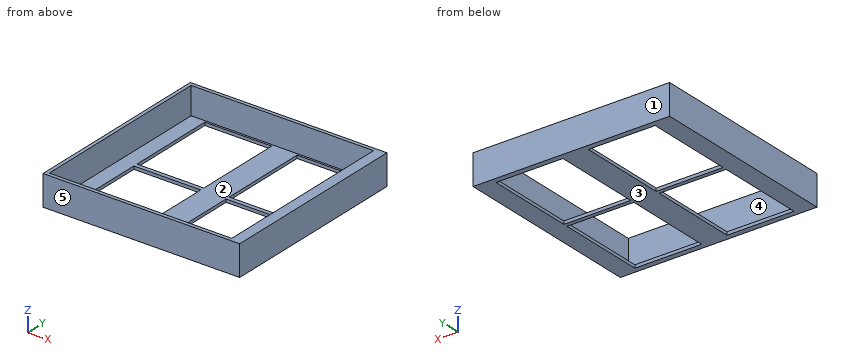
from build123d import *

# Parameters (mm, degrees)
SKETCH_W                        = 194
SKETCH_H                        = 191
PAD_DEPTH                       = 30
SKETCH001_W                     = 180
SKETCH001_H                     = 184
POCKET_DEPTH                    = 27
SKETCH002_W                     = 66
SKETCH002_H                     = 88
POCKET001_DEPTH                 = 5
SKETCH002_LINEARPATTERN_2_W     = 66
SKETCH002_LINEARPATTERN_2_H     = 88
POCKET001_LINEARPATTERN_2_DEPTH = 5
LINEARPATTERN001_COUNT          = 2
LINEARPATTERN001_PITCH          = 92


with BuildPart() as part:
    # Sketch → Pad (new body)
    with BuildSketch(Plane.XY):
        with Locations((97, 95.5)):
            Rectangle(SKETCH_W, SKETCH_H)
    extrude(amount=PAD_DEPTH)

    # Sketch001 (on Face6 of Pad) → Pocket (cut)
    with BuildSketch(Plane.XY.offset(30)):
        with Locations((93.5, 95.5)):
            Rectangle(SKETCH001_W, SKETCH001_H)
    extrude(amount=-POCKET_DEPTH, mode=Mode.SUBTRACT)

    # Sketch002 (on Face11 of Pocket) → Pocket001 (cut)
    with BuildSketch(Plane.XY.offset(3)):
        with Locations((51.5, 141.5)):
            Rectangle(SKETCH002_W, SKETCH002_H)
    pocket001 = extrude(amount=-POCKET001_DEPTH, mode=Mode.SUBTRACT)

    # Sketch002 LinearPattern 2 → Pocket001 LinearPattern 2 (cut)
    with BuildSketch(Plane(origin=(91, 0, 3), x_dir=(1, 0, 0), z_dir=(0, 0, 1))):
        with Locations((51.5, 141.5)):
            Rectangle(SKETCH002_LINEARPATTERN_2_W, SKETCH002_LINEARPATTERN_2_H)
    pocket001_linearpattern_2 = extrude(amount=-POCKET001_LINEARPATTERN_2_DEPTH, mode=Mode.SUBTRACT)

    # LinearPattern001: Pocket001, Pocket001 LinearPattern 2 ×2
    with Locations(*[(0, -i * LINEARPATTERN001_PITCH, 0) for i in range(1, LINEARPATTERN001_COUNT)]):
        add(pocket001, mode=Mode.SUBTRACT)
        add(pocket001_linearpattern_2, mode=Mode.SUBTRACT)


solid = part.part
Check sheet for the modelled part. Datum: model origin and axes. Units: mm. Face numbers are marked on the shaded views. A direction names the side the tool comes from. Round coordinates to 2 decimals unless told otherwise and drop trailing zeros. Write each loop counter-clockwise with the first axis right and the second up, starting at its lowest first coordinate (ties: lowest second). Pieces come first, ordered by that corner, then holes. Notation, with made-up numbers: (75.25, -19) -> (121.25, -19) arc R21 cw to (121.25, 7) -> close; hole circle Ø7 at (81.25, -12). An arc over 180 degrees is marked (long way). Answer as CSV lines item,"result". Start each with the question number.
1) Release check for a two-part mould opening along Y. For the marked faces 1, 2 and 3 record: pulls with the +Y half, pulls with the -Y half, needs draft (parallel to the pull), parting line crosses it, or undercut.
2) Material ranges on line 1 (X direction, y = 118, z = 20.75); line 2 (Y direction, x = 158, z = 6); line 3 (Z direction, x = 179.5, y = 67), recorded low to high. Write a range as from..to.
3) Tool access check on the marked faces 4 and 5. Record the directions out of +Z, -Z, +X, -X, +Y, -Y that give a thin tool (end or side, any length) a straight path to the whole face; none if there is none.
4) Section check B-B on x = 75. Enter the section's corners in (y, z), and give its area (3 significant figures).
5) Section check C-C on z = 6.25. Enter the section's corners in (x, y).
6) Section check A-A on y = 101. Enter the section's corners in (x, z), and give its area (3 significant figures).
Found:
1,face 1,"pulls with the +Y half"
1,face 2,"undercut"
1,face 3,"needs draft"
2,line 1,"x = 0..3.5, 183.5..194"
2,line 2,"y = 0..3.5, 187.5..191"
2,line 3,"z = 0..3"
3,face 4,"+Z"
3,face 5,"+Z, -Z, +X, -X, -Y"
4,outline,"(0, 0) -> (5.5, 0) -> (5.5, 3) -> (3.5, 3) -> (3.5, 30) -> (0, 30) -> close; (93.5, 0) -> (97.5, 0) -> (97.5, 3) -> (93.5, 3) -> close; (185.5, 0) -> (191, 0) -> (191, 30) -> (187.5, 30) -> (187.5, 3) -> (185.5, 3) -> close"
4,area,"234 mm^2"
5,outline,"(0, 0) -> (194, 0) -> (194, 191) -> (0, 191) -> close; hole (3.5, 3.5) -> (183.5, 3.5) -> (183.5, 187.5) -> (3.5, 187.5) -> close"
6,outline,"(0, 0) -> (18.5, 0) -> (18.5, 3) -> (3.5, 3) -> (3.5, 30) -> (0, 30) -> close; (84.5, 0) -> (109.5, 0) -> (109.5, 3) -> (84.5, 3) -> close; (175.5, 0) -> (194, 0) -> (194, 30) -> (183.5, 30) -> (183.5, 3) -> (175.5, 3) -> close"
6,area,"564 mm^2"
